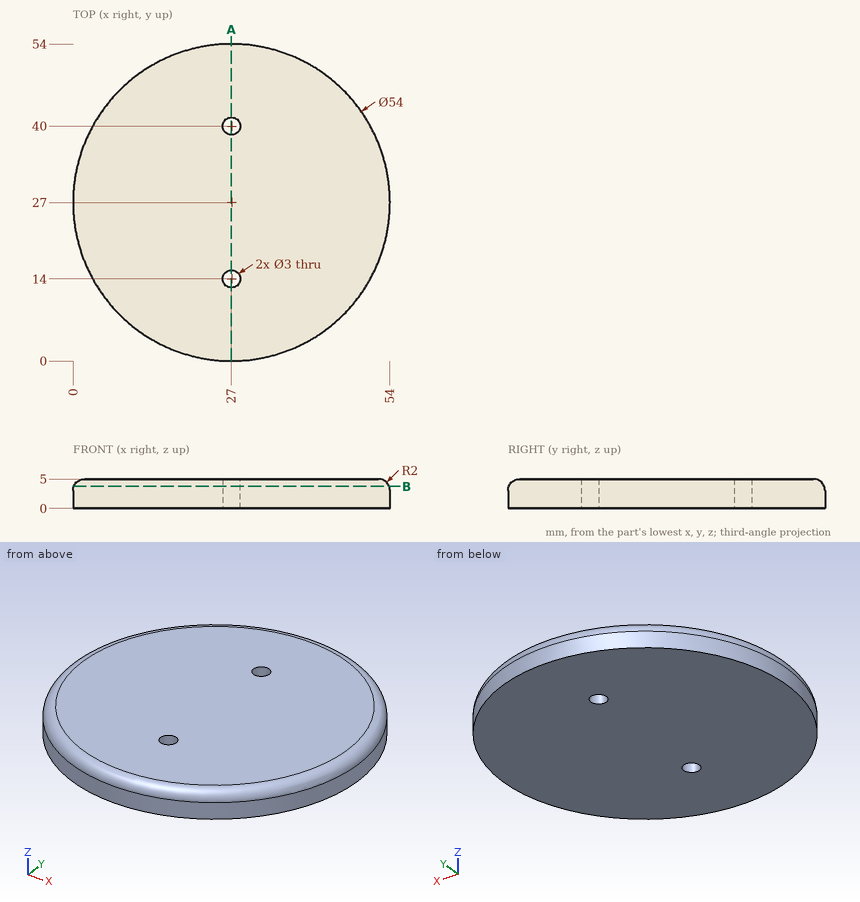
Verification items for this drawing (mm, ordinates from the low corner). Give positions to 0.01 mm unless a question says otherwise; leave off trailing zeros. Write each loop counter-clockwise with the first axis right and the second up, starting at its lowest first coordinate (ties: lowest second). Pieces come first, ordered by that corner, then holes. Notation, with made-up numbers: (-16.5, 73.25) - (10.5, 73.25) arc R28 cw to (10.5, 106.25) - close; hole circle Ø10 at (-9.5, -24). An arc over 180 degrees is marked (long way). Answer as a JSON object with one key per item and string values. Group by question number.
1) Depth check by flat-ended pin: P1, Ø2, axis at x = 36.5, z = 4.5, coming from the +Y side; P2, Ø1.5, axis at x = 19.5, z = 3, coming from the +Y side; P3, Ø2.5, axis at x = 27, y = 40, coming from the -Z side; P4, Ø3, axis at x = 25.5, z = 1.5, coming from the -Y side. Enter the tip coordinate at first touch or a pass-through.
2) Thickness scan on probe 1 along Y at (x, z) = (27, 2.15); probe 2 along Y at (x, z) = (27, 3.9); probe 3 along X at (y, z) = (12, 2.45). Record the ranges inside material, lowest first. Write a range as from..to.
3) Sectioned sample at A-A (x = 27). Give the number of separate pieces and of enclosed holes in the cut face, then the cut area to 3 significant figures.
4) Sectioned sample at B-B (z = 3.75). Record the cut outline in (x, y).
Geometry results:
{
 "1": {"P1": "stops at y = 52.36", "P2": "stops at y = 53.14", "P3": "passes through", "P4": "stops at y = 0"},
 "2": {"probe 1": "y = 0..12.5, 15.5..38.5, 41.5..54", "probe 2": "y = 0.21..12.5, 15.5..38.5, 41.5..53.79", "probe 3": "x = 4.55..49.45"},
 "3": {"separate pieces": "3", "enclosed holes": "0", "area": "238 mm^2"},
 "4": {"outline": "circle Ø53.71 at (27, 27); hole circle Ø3 at (27, 14); hole circle Ø3 at (27, 40)"}
}
